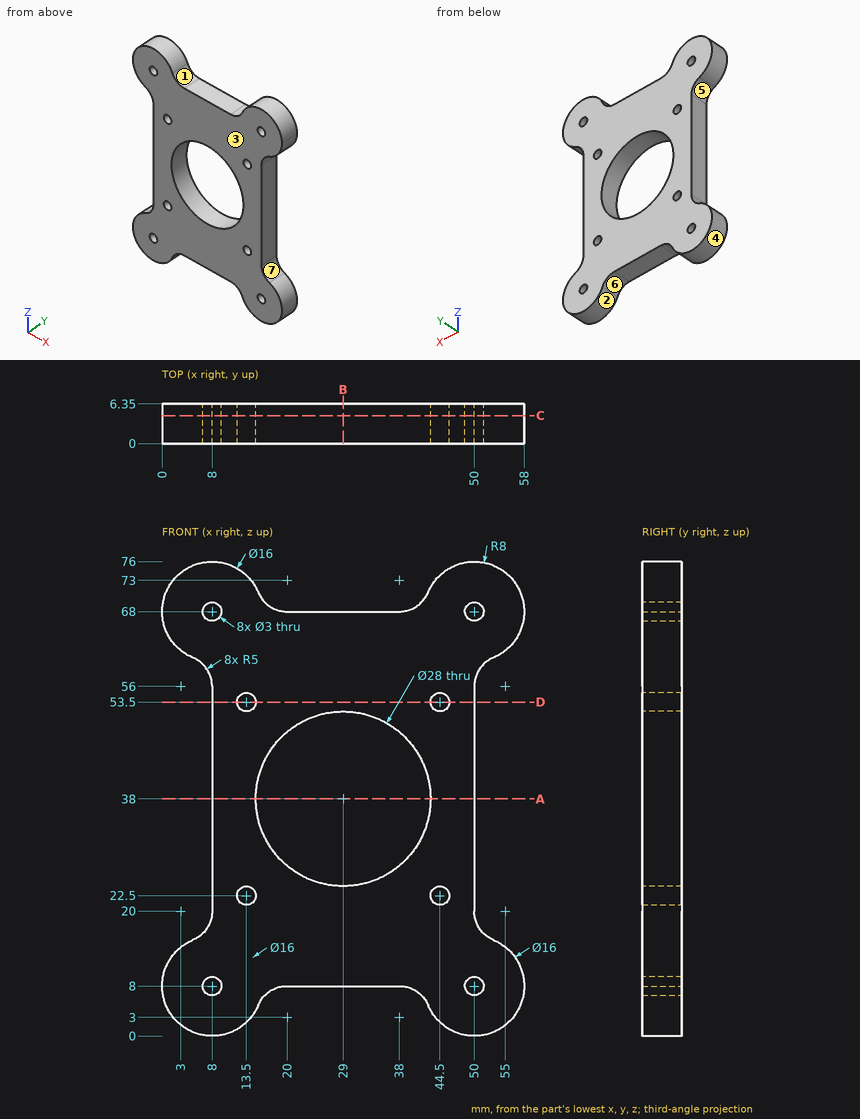
Job drawing, mm, ordinate dimensions from the low corner. One solid piece. A direction names the side the tool comes from. Coordinates: 2 decimals unless noted, no trailing zeros. Loops run counter-clockwise (first coordinate to the right, second up) from the corner with the lowest first, then second, coordinate; pieces in that order, holes last. Notation, with made-up numbers: (-31, -10.75) - (25, -10.75) arc R9 cw to (25, 6.25) - close; hole circle Ø1 at (67, -29.5). An arc over 180 degrees is marked (long way). Answer as a JSON object with one key per item and string values. Group by question number.
(1) Cut at C-C (y = 4.5). State how many separate pieces and enclosed holes the cut face has, then the cut area to 3 significant figures.
(2) Flat gauge pins, fed straight in: pin 1 (1.9 mm diameter, centred on x = 24.5, y = 2.5, fed in from -Z); pin 2 (3 mm diameter, centred on y = 5, z = 42, fed in from -X); pin 3 (1.9 mm diameter, centred on y = 4.5, z = 39, fed in from +X). Where does each tip first touch, or does it go through?
(3) Cut at D-D (z = 53.5). Give the cut face in (x, y).
(4) Two-plate mould, pull along Z, no slides. Class the marked faces 1, 2 and 3: released by +Z, released by -Z, zero draft, split by the parting line, or undercut.
(5) Probe line 1 along X through (y, z) = (2.75, 22.5); line 2 along Z through (x, y) = (51, 5.25); line 3 along X through (y, z) = (2, 23). List the from-to ranges inside material, lowest first.
(6) Cut at A-A (z = 38). Give the cut face in (x, y), then the cut area to 3 significant figures.
(7) Tool access for the marked faces 4, 5, 6 and 7: list every direction of +Z, -Z, +X, -X, +Y, -Y with a clear straight run to the whole face (end or side of a thin tool).
(8) Cut at B-B (x = 29). Give the cut face in (y, z), then the cut area to 3 significant figures.
Geometry says:
{
 "1": {"separate pieces": "1", "enclosed holes": "9", "area": "2,470 mm^2"},
 "2": {"pin 1": "stops at z = 8", "pin 2": "stops at x = 8", "pin 3": "stops at x = 50"},
 "3": {"outline": "(8, 0) - (12, 0) - (12, 6.35) - (8, 6.35) - close; (15, 0) - (43, 0) - (43, 6.35) - (15, 6.35) - close; (46, 0) - (50, 0) - (50, 6.35) - (46, 6.35) - close"},
 "4": {"face 1": "released by +Z", "face 2": "undercut", "face 3": "zero draft"},
 "5": {"line 1": "x = 8 to 12, 15 to 43, 46 to 50", "line 2": "z = 0.06 to 6.88, 9.12 to 17, 59 to 66.88, 69.12 to 75.94", "line 3": "x = 8 to 12.09, 14.91 to 43.09, 45.91 to 50"},
 "6": {"outline": "(8, 0) - (15, 0) - (15, 6.35) - (8, 6.35) - close; (43, 0) - (50, 0) - (50, 6.35) - (43, 6.35) - close", "area": "88.9 mm^2"},
 "7": {"face 4": "+Y, -Y", "face 5": "-X, +Y, -Y", "face 6": "-Z, +Y, -Y", "face 7": "+X, +Y, -Y"},
 "8": {"outline": "(0, 8) - (6.35, 8) - (6.35, 24) - (0, 24) - close; (0, 52) - (6.35, 52) - (6.35, 68) - (0, 68) - close", "area": "203 mm^2"}
}
